Read the model definition and answer for the solid it produces. Units are mm, in the model's axes. Face numbers are marked on the shaded views. Coordinates: 2 decimals unless noted, no trailing zeros. Write each loop counter-clockwise with the first axis right and the second up, starting at its lowest first coordinate (ties: lowest second). Pieces come first, ordered by that corner, then holes.
Item 1: Each of these flat-tipped pins is pushed along its axis until it touches: P1, Ø1, axis at x = -11.5, y = 35, coming from the +Z side; P2, Ø4, axis at x = -16, z = -98.5, coming from the +Y side; P3, Ø6, axis at x = 6, z = -147.5, coming from the +Y side. Where does it stop, or does it pass through?
Item 2: Section A-A (y = 0) is taken. Give the vertices of the cut face in (x, z), then the cut area to 3 significant figures.
Item 3: Determine the mould class of the marked faces 1 and 2 for opening direction Y: released by +Y, released by -Y, zero draft, split by the parting line, or undercut.
Item 4: Section C-C (z = -549) is taken. Give the vertices of the cut face in (x, y).
Item 5: Straight lines are drawn through the part: probe 1 along Z at (x, y) = (18, 49); probe 2 along Y at (x, z) = (-0.5, -334) (3 decimals); probe 3 along Z at (x, y) = (23, 37.5). For each, find the intervals that lie inside material, in ascending order.
from build123d import *

# Parameters (mm, degrees)
F2_R = 5


# Not quite as in the source:
# - a fillet or chamfer that OpenCascade refuses, or shapes differently, is made with other operations: its cross-section is extruded or revolved along the edge and cut away or added


with BuildPart() as f1:
    # F0 (on Front) → F1 (revolve)
    with BuildSketch(Plane.XZ):
        Polygon((0, -800), (0, 0), (-60, 0), (-60, -50), (-40, -50), (-40, -90), (-25, -90), (-25, -800), align=None)
    revolve(axis=Axis((0, 0, -400), (0, 0, -1)))

    # F2
    f2_edges = [f1.edges().sort_by_distance(p)[0] for p in [
        (40, 0, -50),
    ]]
    fillet(f2_edges, radius=F2_R)

    # F3: fillet of radius 40 on 1 edges, made by hand

    # F3_s1 → F3_t2 (revolve)
    with BuildSketch(Plane.XZ):
        with BuildLine():
            ThreePointArc((-40, -90), (-28.9444872454, -103.9044819163), (-25, -121.224989992))
            Line((-25, -121.224989992), (-25, -90))
            Line((-25, -90), (-40, -90))
        make_face()
    revolve(axis=Axis((0, 0, -90), (0, 0, -1)))


solid = f1.part
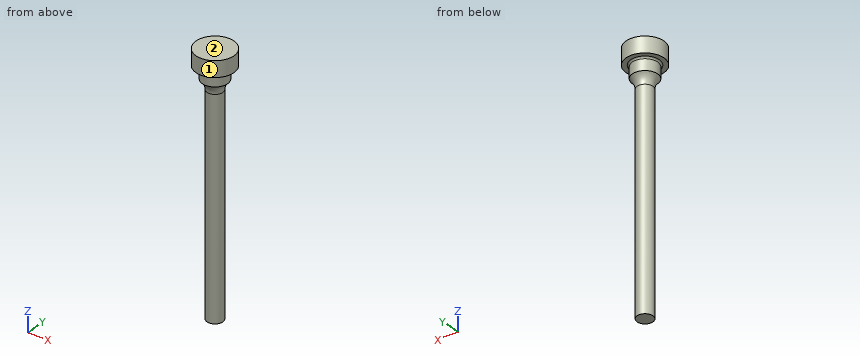
Established:
1. P1: stops at z = 0
1. P2: stops at y = 29.78
1. P3: stops at y = 24.82
2. outline: (-60, -50) - (-45, -50) arc R5 cw to (-40, -55) - (-40, -90) arc R40 cw to (-25, -121.22) - (-25, -800) - (25, -800) - (25, -121.22) arc R40 cw to (40, -90) - (40, -55) arc R5 cw to (45, -50) - (60, -50) - (60, 0) - (-60, 0) - close
2. area: 45,000 mm2
3. face 1: split by the parting line
3. face 2: zero draft
4. outline: circle Ø50 at (0, 0)
5. probe 1: z = -50 to 0
5. probe 2: y = -24.995 to 24.995
5. probe 3: z = -50.1 to 0
